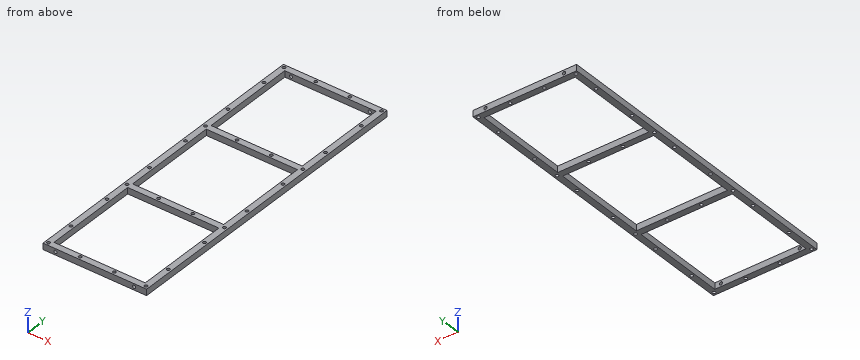
from build123d import *

# Parameters (mm, degrees)
SKETCH1_W           = 100
SKETCH1_H           = 300
SKETCH1_W_2         = 88
SKETCH1_H_2         = 92
BOSS_EXTRUDE1_DEPTH = 6
SKETCH2_R           = 1.5
CUT_EXTRUDE1_DEPTH  = 6
SKETCH3_R           = 1.5
CUT_EXTRUDE2_DEPTH  = 10
SKETCH4_R           = 1.5
CUT_EXTRUDE5_DEPTH  = 10


with BuildPart() as part:
    # Sketch1 → Boss-Extrude1 (new body)
    with BuildSketch(Plane.XY):
        Rectangle(SKETCH1_W, SKETCH1_H)
        with Locations((0, 98)):
            Rectangle(SKETCH1_W_2, SKETCH1_H_2, mode=Mode.SUBTRACT)
        with Locations((0, -98)):
            Rectangle(SKETCH1_W_2, SKETCH1_H_2, mode=Mode.SUBTRACT)
        Rectangle(SKETCH1_W_2, SKETCH1_H_2, mode=Mode.SUBTRACT)
    extrude(amount=BOSS_EXTRUDE1_DEPTH)

    # Sketch2 → Cut-Extrude1 (cut)
    with BuildSketch(Plane.XY.offset(6)):
        with Locations((-47, 147)):
            Circle(SKETCH2_R)
        with Locations((47, 147)):
            Circle(SKETCH2_R)
        with Locations((47, 49)):
            Circle(SKETCH2_R)
        with Locations((47, -49)):
            Circle(SKETCH2_R)
        with Locations((47, -147)):
            Circle(SKETCH2_R)
        with Locations((-47, 49)):
            Circle(SKETCH2_R)
        with Locations((-47, -49)):
            Circle(SKETCH2_R)
        with Locations((-47, -147)):
            Circle(SKETCH2_R)
    extrude(amount=-CUT_EXTRUDE1_DEPTH, mode=Mode.SUBTRACT)

    # Sketch3 → Cut-Extrude2 (cut)
    with BuildSketch(Plane.XY.offset(6)):
        with Locations((-47, -21)):
            Circle(SKETCH3_R)
        with Locations((-16.5, -49)):
            Circle(SKETCH3_R)
        with Locations((-47, -74)):
            Circle(SKETCH3_R)
        with Locations((-47, -119)):
            Circle(SKETCH3_R)
        with Locations((-16.5, -147)):
            Circle(SKETCH3_R)
        with Locations((16.5, -147)):
            Circle(SKETCH3_R)
        with Locations((47, -119)):
            Circle(SKETCH3_R)
        with Locations((47, -74)):
            Circle(SKETCH3_R)
        with Locations((16.5, -49)):
            Circle(SKETCH3_R)
        with Locations((47, -21)):
            Circle(SKETCH3_R)
        with Locations((47, 77)):
            Circle(SKETCH3_R)
        with Locations((16.5, 49)):
            Circle(SKETCH3_R)
        with Locations((-16.5, 147)):
            Circle(SKETCH3_R)
        with Locations((-47, 122)):
            Circle(SKETCH3_R)
        with Locations((16.5, 147)):
            Circle(SKETCH3_R)
        with Locations((-47, 77)):
            Circle(SKETCH3_R)
        with Locations((-16.5, 49)):
            Circle(SKETCH3_R)
        with Locations((-47, 24)):
            Circle(SKETCH3_R)
        with Locations((47, 24)):
            Circle(SKETCH3_R)
        with Locations((47, 122)):
            Circle(SKETCH3_R)
    extrude(amount=-CUT_EXTRUDE2_DEPTH, mode=Mode.SUBTRACT)

    # Sketch4 → Cut-Extrude5 (cut)
    with BuildSketch(Plane(origin=(0, 150, 0), x_dir=(1, 0, 0), z_dir=(0, 1, 0))):
        with Locations(Location((-38, -3, 0), (0, 0, 270))):
            Circle(SKETCH4_R)
        with Locations(Location((38, -3, 0), (0, 0, 90))):
            Circle(SKETCH4_R)
    cut_extrude5 = extrude(amount=-CUT_EXTRUDE5_DEPTH, mode=Mode.SUBTRACT)

    # Mirror1: Cut-Extrude5 across plane
    add(cut_extrude5.mirror(Plane.ZX), mode=Mode.SUBTRACT)


solid = part.part
Can you work these out from the model? Positions are in its coordinate system, mm. Coordinates: 2 decimals unless noted, no trailing zeros. Loops run counter-clockwise (first coordinate to the right, second up) from the corner with the lowest first, then second, coordinate; pieces in that order, holes last. Notation, with made-up numbers: (-7, -25.75) - (7, -25.75) arc R17 ccw to (7, 7.25) - close; hole circle Ø5 at (36, 89). An arc over 180 degrees is marked (long way). Put each result on its own line as item: value. Start each with the question number.
Item 1: Suppose I cut it at B-B (y = -113). Please give me the cut outline in (x, z).
Item 2: If I drill on line 1 along Y through (x, z) = (-33.5, 3.5); line 2 along X through (y, z) = (77, 4.4); line 3 along X through (y, z) = (-104.5, 2.65), over which ranges is the centre line in solid material (lowest first)?
Item 3: Suppose I cut it at A-A (x = 11). Please give me the cut outline in (y, z), and give its area (3 significant figures).
Item 4: Suppose I cut it at C-C (z = 2.4). State how many separate pieces and enclosed holes the cut face has, and give its area (3 significant figures).
Item 5: For pin 1 (3.5 mm diameter, centred on x = 47, y = -21, fed in from +Z); pin 2 (12 mm diameter, centred on x = 11.5, y = 36, fed in from -Z); pin 3 (1.8 mm diameter, centred on x = 38, z = 3, fed in from +Y), each with a flat end and sliding along its axis, tell me the tip position at first contact or that it passes through.
Here are the results:
1. outline: (-50, 0) - (-44, 0) - (-44, 6) - (-50, 6) - close; (44, 0) - (50, 0) - (50, 6) - (44, 6) - close
2. line 1: -150 to -144, -52 to -46, 46 to 52, 144 to 150
2. line 2: -50 to -48.5, -45.5 to -44, 44 to 45.5, 48.5 to 50
2. line 3: -50 to -44, 44 to 50
3. outline: (-150, 0) - (-144, 0) - (-144, 6) - (-150, 6) - close; (-52, 0) - (-46, 0) - (-46, 6) - (-52, 6) - close; (46, 0) - (52, 0) - (52, 6) - (46, 6) - close; (144, 0) - (150, 0) - (150, 6) - (144, 6) - close
3. area: 144 mm²
4. separate pieces: 3
4. enclosed holes: 29
4. area: 5,450 mm²
5. pin 1: z = 6
5. pin 2: through
5. pin 3: y = 52
